The listing builds one solid part. Answer for the finished solid, in the listing's coordinates (mm). Give positions to 0.01 mm unless a question says otherwise; leave off trailing zeros. Write each loop counter-clockwise with the first axis right and the second up, starting at its lowest first coordinate (ties: lowest second). Pieces come first, ordered by that corner, then holes. Notation, with made-up numbers: (18.5, 89.25) - (45.5, 89.25) arc R29 ccw to (45.5, 114.25) - close; hole circle Ø7 at (-4, 88). An arc over 180 degrees is marked (long way). Write each question's results on one line, items separated by ' | '. Start each with the question number.
Q1. Section C-C (z = 1.25) is taken. Determine the outline of the cut face in (x, y), plus the area to 3 significant figures.
Q2. Flat-ended cylindrical pins translate along their axes: pin 1 Ø8 at (x, y) = (10, -9.5) entering from +Z; pin 2 Ø1 at (x, y) = (-2.5, -10) entering from +Z; pin 3 Ø3 at (y, z) = (-11, 1.5) entering from -X. Find the tip coordinate at first contact, or state that the pin passes through.
Q3. Section A-A (y = -1.5) is taken. Determine the outline of the cut face in (x, z).
Q4. Find the intervals of material crossed by probe 1 along X at (y, z) = (-14.75, 3.25); probe 2 along Z at (x, y) = (-6.5, -6.5); probe 3 along Z at (x, y) = (9.25, -7.5), in increasing order.
Q5. Section B-B (x = 0.75) is taken. Determine the outline of the cut face in (y, z).
```python
from build123d import *

# Parameters (mm, degrees)
F0_W     = 25.4
F0_H     = 11.6255704415
F1_DEPTH = 25.4
F3_DEPTH = 25.401


with BuildPart() as f1:
    # F0 (on Front) → F1 (new body)
    with BuildSketch(Plane.XZ):
        Rectangle(F0_W, F0_H)
    extrude(amount=F1_DEPTH)

    # F2 (on face) → F3 (cut, through all)
    with BuildSketch(Plane.XZ.offset(25.4)):
        with BuildLine():
            Line((-12.7, 5.8127852207), (-12.7, -5.613514744))
            ThreePointArc((-12.7, -5.613514744), (0.2798565548, -0.5667526673), (12.6591933696, 5.8127852207))
            Line((12.6591933696, 5.8127852207), (-12.7, 5.8127852207))
        make_face()
    extrude(amount=-F3_DEPTH, mode=Mode.SUBTRACT)


solid = f1.part
```
Answers below:
1) outline: (4.14, -25.4) - (12.7, -25.4) - (12.7, 0) - (4.14, 0) - close | area: 217 mm2
2) pin 1: stops at z = 5.81 | pin 2: stops at z = -1.57 | pin 3: stops at x = 1.52
3) outline: (-12.7, -5.81) - (12.7, -5.81) - (12.7, 5.81) - (12.66, 5.81) arc R132.67 cw to (-12.7, -5.61) - close
4) probe 1: x = 8.06 to 12.7 | probe 2: z = -5.81 to -3.4 | probe 3: z = -5.81 to 3.89
5) outline: (-25.4, -5.81) - (0, -5.81) - (0, -0.35) - (-25.4, -0.35) - close
